Source: CAD feature listing. Evaluate the final solid. Frame: model axes, mm. Coordinates: 2 decimals unless noted, no trailing zeros. Loops run counter-clockwise (first coordinate to the right, second up) from the corner with the lowest first, then second, coordinate; pieces in that order, holes last. Notation, with made-up numbers: M 74,80.5 L 80,80.5 A28 ccw 80,113.5 Z; hole C 84,18.25 d8. An arc over 180 degrees is marked long. One line per question, with ' | ' between items. Start each with the question number.
1. Section query A-A, the plane y = -29.5. Output: boundary loops of the cut face in (x, z).
2. Pin query (flat end, axial travel): P1, Ø3, axis at x = -146.46, y = -155, coming from the +Z side. Return the tip coordinate at first contact, or that it passes through.
3. Section query C-C, the plane x = -198.5. Output: boundary loops of the cut face in (y, z), and give its area (3 significant figures).
4. Section query D-D, the plane x = -177. Output: boundary loops of the cut face in (y, z), and give its area (3 significant figures).
5. Ray query, probe 1 along Y at (x, z) = (-147.5, 0.75); probe 2 along Y at (x, z) = (-158, 0.2); probe 3 along X at (y, z) = (-125, 0.75). Return the intervals inside material, ascending.
6. Section query B-B, the plane z = 1.4. State how many separate pieces and enclosed holes the cut face has, and give its area (3 significant figures).
```python
from build123d import *

# Parameters (mm, degrees)
SKETCH1_R      = 1.6
EXTRUDE1_DEPTH = 3


with BuildPart() as part:
    # Sketch1 → Extrude1 (new body)
    with BuildSketch(Plane.XY):
        Polygon((-234.458183995, 0), (-162.458183995, -176.470588235), (-142.458183995, -176.470588235), (-142.458183995, 0), (-102.858183995, 0), (-102.858183995, 20), (-102.863553327, 20), (-234.458183995, 20), align=None)
        with Locations((-112.858183995, 10)):
            Circle(SKETCH1_R, mode=Mode.SUBTRACT)
        with Locations((-132.858183995, 10)):
            Circle(SKETCH1_R, mode=Mode.SUBTRACT)
        with Locations((-172.858183995, 10)):
            Circle(SKETCH1_R, mode=Mode.SUBTRACT)
        with Locations((-146.458183995, -45)):
            Circle(SKETCH1_R, mode=Mode.SUBTRACT)
        with Locations((-158.458183995, -45)):
            Circle(SKETCH1_R, mode=Mode.SUBTRACT)
        with Locations((-146.458183995, -15)):
            Circle(SKETCH1_R, mode=Mode.SUBTRACT)
        with Locations((-158.458183995, -15)):
            Circle(SKETCH1_R, mode=Mode.SUBTRACT)
        with Locations((-224.458183995, 10)):
            Circle(SKETCH1_R, mode=Mode.SUBTRACT)
        with Locations((-204.458183995, 10)):
            Circle(SKETCH1_R, mode=Mode.SUBTRACT)
        with Locations((-158.458183995, -125)):
            Circle(SKETCH1_R, mode=Mode.SUBTRACT)
        with Locations((-146.458183995, -125)):
            Circle(SKETCH1_R, mode=Mode.SUBTRACT)
        with Locations((-158.458183995, -155)):
            Circle(SKETCH1_R, mode=Mode.SUBTRACT)
        with Locations((-146.458183995, -155)):
            Circle(SKETCH1_R, mode=Mode.SUBTRACT)
        with BuildLine():
            Line((-209.152667208, 0), (-172.544179417, 0))
            ThreePointArc((-172.544179417, 0), (-170.387933052, -1.244909419), (-170.387933052, -3.734728258))
            Line((-170.387933052, -3.734728258), (-191.838092393, -40.887494067))
            ThreePointArc((-191.838092393, -40.887494067), (-194.163782936, -42.126631048), (-196.299663326, -40.583157071))
            Line((-196.299663326, -40.583157071), (-211.457991776, -3.430391262))
            ThreePointArc((-211.457991776, -3.430391262), (-211.219192406, -1.101052676), (-209.152667208, 0))
        make_face(mode=Mode.SUBTRACT)
        with BuildLine():
            Line((-162.458183995, -41.196152423), (-162.458183995, -108.233623843))
            ThreePointArc((-162.458183995, -108.233623843), (-164.880734742, -111.177524717), (-168.235885568, -109.366926085))
            Line((-168.235885568, -109.366926085), (-184.261936587, -70.087389274))
            ThreePointArc((-184.261936587, -70.087389274), (-184.477279763, -68.749922566), (-184.082311226, -67.454087032))
            Line((-184.082311226, -67.454087032), (-168.056260207, -39.696152423))
            ThreePointArc((-168.056260207, -39.696152423), (-164.68172686, -38.298374944), (-162.458183995, -41.196152423))
        make_face(mode=Mode.SUBTRACT)
    extrude(amount=EXTRUDE1_DEPTH)


solid = part.part
```
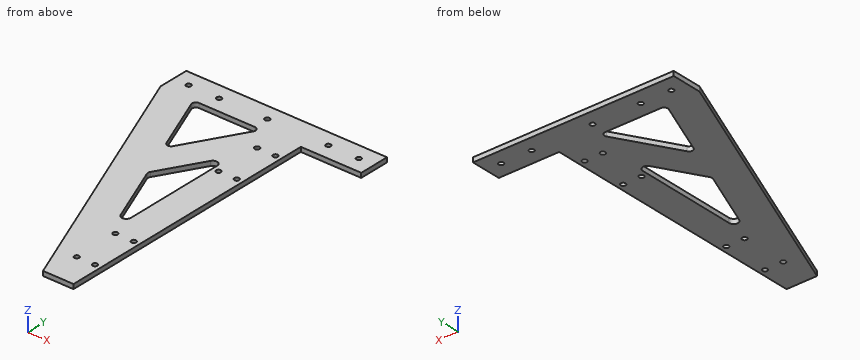
Taken from the geometry:
1) outline: M -222.42,0 L -200.82,0 L -200.82,3 L -222.42,3 Z; M -185.26,0 L -142.46,0 L -142.46,3 L -185.26,3 Z
2) P1: through
3) outline: M -88.13,0 L -35.19,0 L -35.19,3 L -88.13,3 Z; M 0,0 L 20,0 L 20,3 L 0,3 Z | area: 219 mm^2
4) outline: M -140.83,0 L -87.89,0 L -87.89,3 L -140.83,3 Z; M -55.19,0 L -15.19,0 L -15.19,3 L -55.19,3 Z; M 0,0 L 20,0 L 20,3 L 0,3 Z | area: 339 mm^2
5) probe 1: -176.47 to -156.21, -153.79 to -126.21, -123.79 to -46.21, -43.79 to -16.21, -13.79 to 20 | probe 2: -176.47 to -156.53, -153.47 to -126.53, -123.47 to -46.53, -43.47 to -16.53, -13.47 to 20 | probe 3: -183.46 to -160.06, -156.86 to -148.06, -144.86 to -142.46
6) separate pieces: 1 | enclosed holes: 15 | area: 10,400 mm^2
